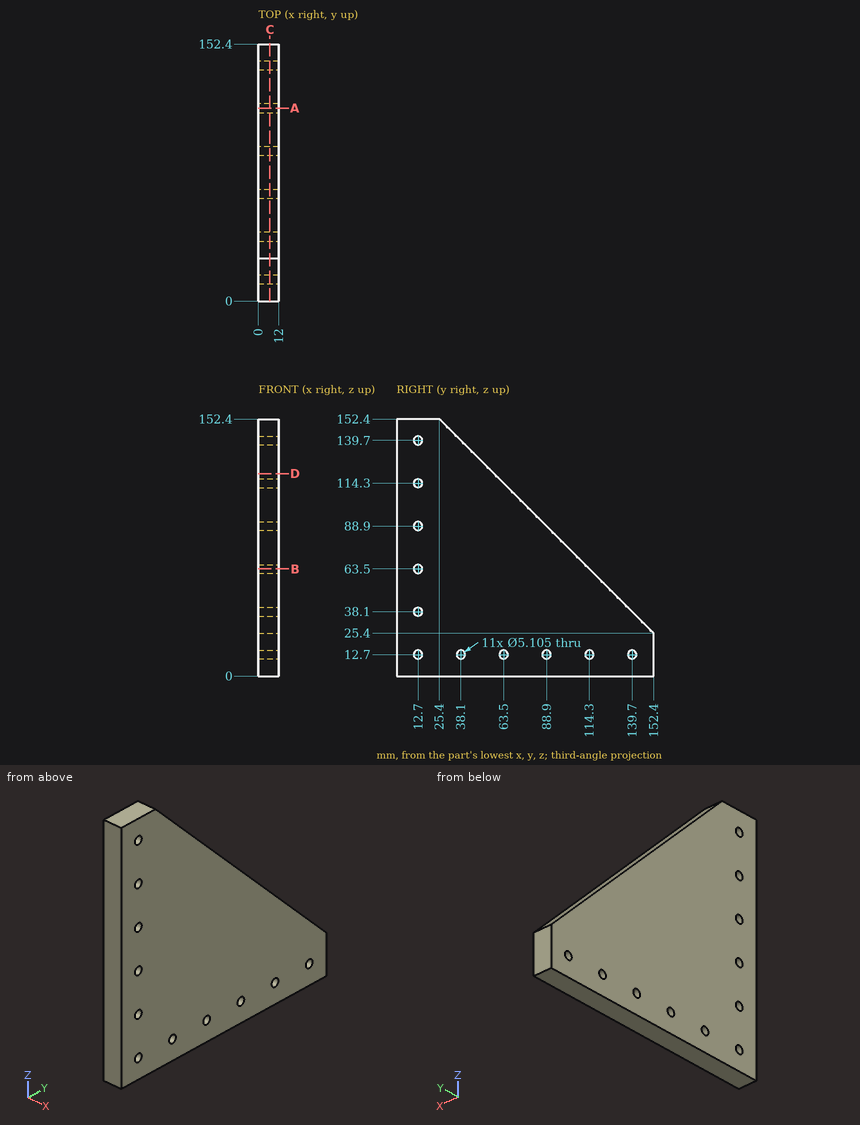
The drawing under review shows one solid part. Ordinate dimensions are in mm from its lowest x, y, z. Give positions to 0.01 mm unless a question says otherwise; leave off trailing zeros. Loops run counter-clockwise (first coordinate to the right, second up) from the corner with the lowest first, then second, coordinate; pieces in that order, holes last. Notation, with made-up numbers: M -27.5,29 L 8.5,29 A15 ccw 8.5,58 Z; hole C -24,-5.5 d9. An arc over 180 degrees is marked long. Return JSON: item names as keys, results as strings. Group by question number.
Item 1: We need section C-C (x = 6.75). Give the number of separate pieces and of enclosed holes in the cut face, and give its area (3 significant figures).
Item 2: Insertion check: pin 1 Ø1 at (x, y) = (3, 75) entering from +Z; pin 2 Ø1 at (x, z) = (1.5, 119) entering from +Y; pin 3 Ø1 at (x, y) = (3, 125) entering from +Z. Each pin has a flat end and moves straight along its axis. Give the tip position at first contact, or say it passes through.
Item 3: We need section D-D (z = 120). Give the boundary of the cut face in (x, y).
Item 4: We need section A-A (y = 114.3). Give the boundary of the cut face in (x, z).
Item 5: For probe 1 along Z at (x, y) = (6.5, 39.5) (1 decimal); probe 2 along Z at (x, y) = (3.5, 88.9) (1 decimal); probe 3 along Y at (x, z) = (11, 122.5), list the stretches that pass through material, from the lowest coordinate up.
Item 6: We need section B-B (z = 63.5). Give the boundary of the cut face in (x, y).
Output:
{
 "1": {"separate pieces": "1", "enclosed holes": "11", "area": "14,900 mm^2"},
 "2": {"pin 1": "stops at z = 103.3", "pin 2": "stops at y = 59.3", "pin 3": "stops at z = 53.3"},
 "3": {"outline": "M 0,0 L 12,0 L 12,57.8 L 0,57.8 Z"},
 "4": {"outline": "M 0,0 L 12,0 L 12,10.15 L 0,10.15 Z; M 0,15.25 L 12,15.25 L 12,63.5 L 0,63.5 Z"},
 "5": {"probe 1": "z = 0 to 10.6, 14.8 to 138.3", "probe 2": "z = 0 to 10.1, 15.3 to 88.9", "probe 3": "y = 0 to 55.3"},
 "6": {"outline": "M 0,0 L 12,0 L 12,10.15 L 0,10.15 Z; M 0,15.25 L 12,15.25 L 12,114.3 L 0,114.3 Z"}
}
